from build123d import *

# Parameters (mm, degrees)
SKETCH1_W           = 43.7261
SKETCH1_H           = 38.2651
BOSS_EXTRUDE1_DEPTH = 3.4544
SKETCH2_W           = 9.3218
SKETCH2_H           = 25.8064
BOSS_EXTRUDE2_DEPTH = 5.334
SKETCH3_W           = 0.635
SKETCH3_H           = 21.463
BOSS_EXTRUDE3_DEPTH = 5.08
SKETCH4_R           = 1.0922
CUT_EXTRUDE1_DEPTH  = 5.08
SKETCH5_W           = 19.9644
SKETCH5_H           = 26.3144
BOSS_EXTRUDE4_DEPTH = 3.9624
SKETCH6_R           = 6.985
BOSS_EXTRUDE5_DEPTH = 6.5024
SKETCH7_R           = 1.524
BOSS_EXTRUDE6_DEPTH = 3.6195


with BuildPart() as part:
    # Sketch1 → Boss-Extrude1 (new body)
    with BuildSketch(Plane.XY):
        with Locations((-21.86305, 19.13255)):
            Rectangle(SKETCH1_W, SKETCH1_H)
    extrude(amount=BOSS_EXTRUDE1_DEPTH)

    # Sketch2 → Boss-Extrude2 (add)
    with BuildSketch(Plane(origin=(0, 0, 0), x_dir=(-1, 0, 0), z_dir=(0, 0, -1))):
        with Locations((-1.0033, 11.7348)):
            Rectangle(SKETCH2_W, SKETCH2_H)
    extrude(amount=BOSS_EXTRUDE2_DEPTH)

    # Sketch3 → Boss-Extrude3 (add)
    with BuildSketch(Plane.XY):
        with Locations((4.3307, 11.5951)):
            Rectangle(SKETCH3_W, SKETCH3_H)
    extrude(amount=BOSS_EXTRUDE3_DEPTH)

    # Sketch4 → Cut-Extrude1 (cut)
    with BuildSketch(Plane(origin=(0, 0, 0), x_dir=(-1, 0, 0), z_dir=(0, 0, -1))):
        with Locations((41.2623, 35.8013)):
            Circle(SKETCH4_R)
        with Locations((41.2623, 2.4638)):
            Circle(SKETCH4_R)
        with Locations((8.128, 2.4638)):
            Circle(SKETCH4_R)
        with Locations((8.128, 35.8013)):
            Circle(SKETCH4_R)
    extrude(amount=-CUT_EXTRUDE1_DEPTH, mode=Mode.SUBTRACT)

    # Sketch5 → Boss-Extrude4 (add)
    with BuildSketch(Plane.XY.offset(3.4544)):
        with Locations((-24.5999, 19.558)):
            Rectangle(SKETCH5_W, SKETCH5_H)
    extrude(amount=BOSS_EXTRUDE4_DEPTH)

    # Sketch6 → Boss-Extrude5 (add)
    with BuildSketch(Plane(origin=(0, 0, 12.7762), x_dir=(-1, 0, 0), z_dir=(0, 0, -1))):
        with Locations((24.5999, 19.558)):
            Circle(SKETCH6_R)
    extrude(amount=BOSS_EXTRUDE5_DEPTH)

    # Sketch7 → Boss-Extrude6 (add)
    with BuildSketch(Plane(origin=(0, 0, 0), x_dir=(-1, 0, 0), z_dir=(0, 0, -1))):
        with Locations((25.4381, 30.0482)):
            Circle(SKETCH7_R)
        with Locations((25.4381, 8.128)):
            Circle(SKETCH7_R)
    extrude(amount=BOSS_EXTRUDE6_DEPTH)


solid = part.part
Verification items for the finished model (mm, model axes). A direction names the side the tool comes from. Coordinates: 2 decimals unless noted, no trailing zeros. Order: outer loops, then holes, each group sorted by start corner. A loop starts at its lowest first (then second) coordinate and runs counter-clockwise, first axis right, second up.
Item 1: Depth check by flat-ended pin: pin 1 (1.2 mm diameter, centred on x = -25.5, z = 6, fed in from -Y); pin 2 (0.5 mm diameter, centred on x = 4.5, z = 3, fed in from +Y); pin 3 (4.5 mm diameter, centred on x = 0.5, y = 6.5, fed in from +Z). Enter the tip coordinate at first touch or a pass-through.
Filled in:
pin 1: stops at y = 6.4
pin 2: stops at y = 22.33
pin 3: stops at z = 3.45
Item 2: Section check D-D, the plane x = -29. Enter the section's corners in (y, z), then the cut area to 3 significant figures.
Filled in:
outline: (0, 0) - (38.27, 0) - (38.27, 3.45) - (32.72, 3.45) - (32.72, 7.42) - (24.98, 7.42) - (24.98, 12.78) - (14.13, 12.78) - (14.13, 7.42) - (6.4, 7.42) - (6.4, 3.45) - (0, 3.45) - close
area: 295 mm2
Item 3: Section check A-A, the plane z = 0.75. Enter the section's corners in (x, y).
Filled in:
outline: (-43.73, 0) - (0, 0) - (0, 38.27) - (-43.73, 38.27) - close; (4.01, 0.86) - (4.65, 0.86) - (4.65, 22.33) - (4.01, 22.33) - close; hole circle Ø2.18 at (-41.26, 2.46); hole circle Ø2.18 at (-41.26, 35.8); hole circle Ø2.18 at (-8.13, 2.46); hole circle Ø2.18 at (-8.13, 35.8)
Item 4: Section check C-C, the plane x = -16. Enter the section's corners in (y, z).
Filled in:
outline: (0, 0) - (38.27, 0) - (38.27, 3.45) - (32.72, 3.45) - (32.72, 7.42) - (6.4, 7.42) - (6.4, 3.45) - (0, 3.45) - close
Item 5: Section check B-B, the plane y = 11. Enter the section's corners in (x, z), then the cut area to 3 significant figures.
Filled in:
outline: (-43.73, 0) - (-3.66, 0) - (-3.66, -5.33) - (5.66, -5.33) - (5.66, 0) - (4.65, 0) - (4.65, 5.08) - (4.01, 5.08) - (4.01, 0) - (0, 0) - (0, 3.45) - (-14.62, 3.45) - (-14.62, 7.42) - (-34.58, 7.42) - (-34.58, 3.45) - (-43.73, 3.45) - close
area: 283 mm2
Item 6: Material ranges on L1, parallel to X at y = 10, z = 1.5; L2, parallel to Z at x = -41, y = 1; L3, parallel to Z at x = -15, y = 21, recorded low to high.
Filled in:
L1: x = -43.73 to 0, 4.01 to 4.65
L2: z = 0 to 3.45
L3: z = 0 to 7.42
Item 7: Release check for a two-part mould opening along Y. For faces 6 (the face through (-25, 32.715, 5)), 7 (the face through (-43.726, 19, 2)), 8 (the face through (-9.14, 2.05, 1.7)) record: +Y half, -Y half, draft (parallel to the pull), parting line (faces both ways), or undercut.
Filled in:
face 6: +Y half
face 7: draft
face 8: undercut
Item 8: Access from +Z, -Z, +X, -X, +Y, -Y to the whole of each face (thin tool, end or side, straight path). Record for faces 1 (the face through (0, 19, 2)), 2 (the face through (1, 24.638, -3)), 3 (the face through (-34.582, 19, 5)), 4 (the face through (-25, 6.401, 5)), 5 (the face through (-26.846, 29.464, -1.784)).
Filled in:
face 1: +Z, +Y, -Y
face 2: -Z, +X, -X, +Y
face 3: +Z, -X, +Y, -Y
face 4: +Z, -X, -Y
face 5: -Z
